from build123d import *

# Parameters (mm, degrees)
BOSS_EXTRUDE1_DEPTH      = 4.5
FILLET1_R                = 2
BOSS_EXTRUDE2_DEPTH      = 8
M4_CLEARANCE_HOLE1_D     = 4.5
M4_CLEARANCE_HOLE1_DEPTH = 12.4
M4_CLEARANCE_HOLE1_TIP   = 1.351936393
SKETCH9_W                = 9
SKETCH9_H                = 3.5
BOSS_EXTRUDE3_DEPTH      = 2.5
SKETCH10_W               = 17
SKETCH10_H               = 3.5
BOSS_EXTRUDE4_DEPTH      = 2.5
SKETCH11_W               = 5
SKETCH11_H               = 2
CUT_EXTRUDE1_DEPTH       = 26.8
FILLET2_R                = 1


with BuildPart() as part:
    # Sketch3 → Boss-Extrude1 (new body, symmetric)
    with BuildSketch(Plane(origin=(0, 0, 0), x_dir=(0, 0, -1), z_dir=(1, 0, 0))):
        with BuildLine():
            Line((-23.3, -14.200000018), (-23.3, -6.5))
            Line((-23.3, -6.5), (-5, -6.5))
            Line((-5, -6.5), (-5, -14.200000018))
            Line((-5, -14.200000018), (-2.5, -14.200000018))
            Line((-2.5, -14.200000018), (-2.5, -12.5))
            ThreePointArc((-2.5, -12.5), (-1.767766953, -10.732233047), (0, -10))
            Line((0, -10), (0, 10))
            Line((0, 10), (-4, 10))
            Line((-4, 10), (-4, -4))
            Line((-4, -4), (-25.8, -4))
            Line((-25.8, -4), (-25.8, -14.200000018))
            Line((-25.8, -14.200000018), (-23.3, -14.200000018))
        make_face()
    extrude(amount=BOSS_EXTRUDE1_DEPTH, both=True)

    # Fillet1
    fillet1_edges = [part.edges().sort_by_distance(p)[0] for p in [
        (0, -10, 0),
        (0, -4, 25.8),
    ]]
    fillet(fillet1_edges, radius=FILLET1_R)

    # Sketch8 → Boss-Extrude2 (add)
    with BuildSketch(Plane(origin=(4.5, 0, 0), x_dir=(0, 0, -1), z_dir=(1, 0, 0))):
        with BuildLine():
            Line((-4, -4), (-5, -6.5))
            Line((-5, -6.5), (-5, -14.200000018))
            Line((-5, -14.200000018), (-2.5, -14.200000018))
            Line((-2.5, -14.200000018), (-2.5, -12.5))
            ThreePointArc((-2.5, -12.5), (-2.124591464, -11.182384308), (-1.111111111, -10.260483959))
            ThreePointArc((-1.111111111, -10.260483959), (-0.300326829, -9.522963679), (0, -8.468871126))
            Line((0, -8.468871126), (0, 10))
            Line((0, 10), (-4, 10))
            Line((-4, 10), (-4, -4))
        make_face()
    extrude(amount=BOSS_EXTRUDE2_DEPTH)

    # M4 Clearance Hole1
    with Locations(Plane(origin=(0, 0, 0), x_dir=(1, 0, 0), z_dir=(0, 0, -1))):
        with Locations((4, 0)):
            Hole(M4_CLEARANCE_HOLE1_D / 2, depth=M4_CLEARANCE_HOLE1_DEPTH)
            with Locations((0, 0, -(M4_CLEARANCE_HOLE1_DEPTH + M4_CLEARANCE_HOLE1_TIP / 2))):  # 118° drill point
                Cone(0, M4_CLEARANCE_HOLE1_D / 2, M4_CLEARANCE_HOLE1_TIP, mode=Mode.SUBTRACT)

    # Sketch9 → Boss-Extrude3 (add)
    with BuildSketch(Plane.XY.offset(25.8)):
        with Locations((0, -15.950000018)):
            Rectangle(SKETCH9_W, SKETCH9_H)
    extrude(amount=-BOSS_EXTRUDE3_DEPTH)

    # Sketch10 → Boss-Extrude4 (add)
    with BuildSketch(Plane.XY.offset(5)):
        with Locations((4, -15.950000018)):
            Rectangle(SKETCH10_W, SKETCH10_H)
    extrude(amount=-BOSS_EXTRUDE4_DEPTH)

    # Sketch11 → Cut-Extrude1 (cut, through all)
    with BuildSketch(Plane.XY.offset(25.8)):
        with Locations((0, -15.200000018)):
            Rectangle(SKETCH11_W, SKETCH11_H)
    extrude(amount=-CUT_EXTRUDE1_DEPTH, mode=Mode.SUBTRACT)

    # Fillet2
    fillet2_edges = [part.edges().sort_by_distance(p)[0] for p in [
        (4, 10, 0),
        (4, 10, 4),
        (0, -17.700000018, 25.8),
        (0, -17.700000018, 23.3),
        (4, -17.700000018, 5),
        (4, -17.700000018, 2.5),
    ]]
    fillet(fillet2_edges, radius=FILLET2_R)


solid = part.part
Model file for the job. Use its own axes, mm. A direction names the side the tool comes from. Give positions to 0.01 mm unless a question says otherwise; leave off trailing zeros. Loops run counter-clockwise (first coordinate to the right, second up) from the corner with the lowest first, then second, coordinate; pieces in that order, holes last. Notation, with made-up numbers: (-35, -31.75) - (13, -31.75) arc R21 ccw to (13, -9.75) - close; hole circle Ø5 at (-31.75, 71.5). An arc over 180 degrees is marked (long way). Use one line per item in the form item = value.
(1) Drill centre lines: L1, parallel to Z at x = 4.25, y = -14.75; L2, parallel to Z at x = 1.75, y = -7.5; L3, parallel to Z at x = -1.25, y = 7. Where is each one in solid material? Low to high.
Determined:
L1 = 2.5 to 5, 23.3 to 25.8
L2 = 0 to 5, 23.3 to 25.8
L3 = 0 to 4
(2) Cut at A-A (y = -8). Give the cut face in (x, z).
Determined:
outline = (-4.5, 0) - (12.5, 0) - (12.5, 5) - (-4.5, 5) - close; (-4.5, 23.3) - (4.5, 23.3) - (4.5, 25.8) - (-4.5, 25.8) - close
(3) Cut at B-B (x = 4). Give the cut face in (y, z), then the cut area to 3 significant figures.
Determined:
outline = (-17.7, 3.5) arc R1 ccw to (-16.7, 2.5) - (-12.5, 2.5) arc R2.5 cw to (-10.26, 1.11) arc R2 ccw to (-8.47, 0) - (-2.25, 0) - (-2.25, 4) - (-4, 4) - (-4, 23.8) arc R2 ccw to (-6, 25.8) - (-16.7, 25.8) arc R1 ccw to (-17.7, 24.8) - (-17.7, 24.3) arc R1 ccw to (-16.7, 23.3) - (-6.5, 23.3) - (-6.5, 5) - (-16.7, 5) arc R1 ccw to (-17.7, 4) - close; (2.25, 0) - (9, 0) arc R1 ccw to (10, 1) - (10, 3) arc R1 ccw to (9, 4) - (2.25, 4) - close
area = 166 mm^2
(4) Cut at D-D (y = 0). Give the cut face in (x, z).
Determined:
outline = (-4.5, 0) - (1.75, 0) - (1.75, 4) - (-4.5, 4) - close; (6.25, 0) - (12.5, 0) - (12.5, 4) - (6.25, 4) - close
(5) 3-axis set-ups, long thin cutter, end or side, ignore diameter. For faces 4 (the face through (0, -4, 14)), 5 (the face through (0, -12, 23.3)), 6 (the face through (-2.5, -15, 25)), 7 (the face through (8.44, -5.23, 4.49)): which of +Z, -Z, +X, -X, +Y, -Y reach the whole face in a straight line?
Determined:
face_4 = +Z, +X, -X, +Y
face_5 = +X, -X, -Y
face_6 = +Z, -Z
face_7 = +Z, +X, +Y
(6) Cut at C-C (x = -3). Give the cut face in (y, z), then the cut area to 3 significant figures.
Determined:
outline = (-17.7, 3.5) arc R1 ccw to (-16.7, 2.5) - (-12.5, 2.5) arc R2.5 cw to (-10.26, 1.11) arc R2 ccw to (-8.47, 0) - (9, 0) arc R1 ccw to (10, 1) - (10, 3) arc R1 ccw to (9, 4) - (-4, 4) - (-4, 23.8) arc R2 ccw to (-6, 25.8) - (-16.7, 25.8) arc R1 ccw to (-17.7, 24.8) - (-17.7, 24.3) arc R1 ccw to (-16.7, 23.3) - (-6.5, 23.3) - (-6.5, 5) - (-16.7, 5) arc R1 ccw to (-17.7, 4) - close
area = 184 mm^2
(7) Pull direction Z, two halves, no side cores. Call faces 1 (the face through (4.119, -17.415, 4.699)), 2 (the face through (3.881, 9.715, 3.699)), 3 (the face through (-4.5, -5, 10)): pulls with the +Z half, pulls with the -Z half, needs draft (parallel to the pull), parting line crosses it, or undercut.
Determined:
face_1 = undercut
face_2 = pulls with the +Z half
face_3 = needs draft
(8) Drop flat-ended pins along their axis: P1, Ø2, axis at x = 4, z = 23, coming from the -Y side; P2, Ø8, axis at x = 5, z = 10.5, coming from the +Y side; P3, Ø2.5, axis at x = 0, y = -11, coming from the -Z side. Give the stop position or say it passes through.
Determined:
P1 = -17.65
P2 = -4
P3 = 0.46
